Geometry check sheet. Reference: the model listing, model coordinates, mm. A direction names the side the tool comes from. Coordinates: 2 decimals unless noted, no trailing zeros. Loops run counter-clockwise (first coordinate to the right, second up) from the corner with the lowest first, then second, coordinate; pieces in that order, holes last.
from build123d import *

# Parameters (mm, degrees)
F0_W     = 304.8
F0_H     = 914.4
F0_W_2   = 266.7
F0_H_2   = 876.3
F1_DEPTH = 114.3
F2_W     = 304.8
F2_H     = 914.4
F3_DEPTH = 19.05
F4_W     = 6.35
F4_H     = 4.445
F5_DEPTH = 95.25


with BuildPart() as f1:
    # F0 (on Front) → F1 (new body)
    with BuildSketch(Plane.XZ):
        Rectangle(F0_W, F0_H)
        Rectangle(F0_W_2, F0_H_2, mode=Mode.SUBTRACT)
    extrude(amount=F1_DEPTH)

    # F2 (on face) → F3 (join)
    with BuildSketch(Plane(origin=(0, 0, 0), x_dir=(-1, 0, 0), z_dir=(0, 1, 0))):
        Rectangle(F2_W, F2_H)
    extrude(amount=-F3_DEPTH)

    # F4 (on face) → F5 (cut)
    with BuildSketch(Plane.XZ.offset(114.3)):
        with Locations((-136.525, 341.822318)):
            Rectangle(F4_W, F4_H)
        with Locations((-136.525, 196.148134)):
            Rectangle(F4_W, F4_H)
        with Locations((-136.525, 31.573584)):
            Rectangle(F4_W, F4_H)
        with Locations((-136.525, -160.389908)):
            Rectangle(F4_W, F4_H)
        with Locations((136.525, 196.148134)):
            Rectangle(F4_W, F4_H)
        with Locations((136.525, 341.822318)):
            Rectangle(F4_W, F4_H)
        with Locations((136.525, -160.389908)):
            Rectangle(F4_W, F4_H)
        with Locations((136.525, 31.573584)):
            Rectangle(F4_W, F4_H)
    extrude(amount=-F5_DEPTH, mode=Mode.SUBTRACT)


solid = f1.part
(1) Scan lines: L1, parallel to Z at x = 90, y = -24; L2, parallel to X at y = -68.5, z = 108; L3, parallel to Z at x = 133.5, y = -55.5. Record each from-to range of solid material in increasing order.
Findings:
L1: z = -457.2 to -438.15, 438.15 to 457.2
L2: x = -152.4 to -133.35, 133.35 to 152.4
L3: z = -457.2 to -162.61, -158.17 to 29.35, 33.8 to 193.93, 198.37 to 339.6, 344.04 to 457.2
(2) Access from +Z, -Z, +X, -X, +Y, -Y to the whole of each face (thin tool, end or side, straight path). Record for faces 5 (the flat face through (-2, 0, 6)), 6 (the flat face through (133.35, -66, -302)).
Findings:
face 5: +Z, -Z, +X, -X, +Y
face 6: -Y
(3) Sectioned sample at A-A on x = 121.5. Record the cut outline in (y, z), and give its area (3 significant figures).
Findings:
outline: (-114.3, -457.2) - (0, -457.2) - (0, 457.2) - (-114.3, 457.2) - (-114.3, 438.15) - (-19.05, 438.15) - (-19.05, -438.15) - (-114.3, -438.15) - close
area: 21,000 mm2
(4) Draft check along X on faces 1 (the flat face through (2, -19.05, 6)), 2 (the flat face through (-152.4, -56, -6)), 3 (the flat face through (-133.35, -66, -302)), 4 (the flat face through (-2, -56, -457.2)). Enter one of: +X half, -X half, draft (parallel to the pull), parting line (faces both ways), or undercut.
Findings:
face 1: undercut
face 2: -X half
face 3: undercut
face 4: draft
(5) Sectioned sample at B-B on z = 126. Record the cut outline in (x, y).
Findings:
outline: (-152.4, -114.3) - (-133.35, -114.3) - (-133.35, -19.05) - (133.35, -19.05) - (133.35, -114.3) - (152.4, -114.3) - (152.4, 0) - (-152.4, 0) - close
(6) Gauge pin test, flat end, axial feed: pin 1 Ø4 at (x, z) = (39, -201.5) entering from -Y. Record the tip position at first contact, or that the pin passes through.
Findings:
pin 1: stops at y = -19.05
